Could you check a few things on this model? Use its own coordinates, in mm. Face numbers are marked on the shaded views. A direction names the side the tool comes from. Round coordinates to 2 decimals unless told otherwise and drop trailing zeros. Loops run counter-clockwise (first coordinate to the right, second up) from the corner with the lowest first, then second, coordinate; pieces in that order, holes last. Notation, with made-up numbers: M 27,11.25 L 78,11.25 A25 cw 78,23.25 Z; hole C 56.25,-19 d3. An arc over 180 degrees is marked long. Answer in a Markdown table with one row per item.
```python
from build123d import *

# Parameters (mm, degrees)
F1_DEPTH = 96
F2_R     = 7.5
F3_DEPTH = 30
F4_R     = 6
F5_DEPTH = 3
F6_R     = 6
F7_DEPTH = 3


with BuildPart() as f1:
    # F0 (on Top) → F1 (new body)
    with BuildSketch(Plane.XY):
        with BuildLine():
            ThreePointArc((0, -10), (-2.928932, -2.928932), (-10, 0))
            Line((-10, 0), (-97, 0))
            ThreePointArc((-97, 0), (-104.071068, -2.928932), (-107, -10))
            Line((-107, -10), (-107, -97))
            ThreePointArc((-107, -97), (-104.071068, -104.071068), (-97, -107))
            Line((-97, -107), (-10, -107))
            ThreePointArc((-10, -107), (-2.928932, -104.071068), (0, -97))
            Line((0, -97), (0, -10))
        make_face()
    extrude(amount=F1_DEPTH)

    # F2 (on face) → F3 (join)
    with BuildSketch(Plane(origin=(0, 0, 0), x_dir=(1, 0, 0), z_dir=(0, 0, -1))):
        with Locations((-53.5, 53.5)):
            Circle(F2_R)
    extrude(amount=F3_DEPTH)

    # F4 (on face) → F5 (cut)
    with BuildSketch(Plane.XY.offset(96)):
        with Locations((-94.5, -94.5)):
            Circle(F4_R)
        with Locations((-94.5, -12.5)):
            Circle(F4_R)
        with Locations((-12.5, -94.5)):
            Circle(F4_R)
        with Locations((-12.5, -12.5)):
            Circle(F4_R)
    extrude(amount=-F5_DEPTH, mode=Mode.SUBTRACT)

    # F6 (on face) → F7 (cut)
    with BuildSketch(Plane(origin=(0, 0, 0), x_dir=(1, 0, 0), z_dir=(0, 0, -1))):
        with Locations((-10, 97)):
            Circle(F6_R)
        with Locations((-10, 10)):
            Circle(F6_R)
        with Locations((-97, 97)):
            Circle(F6_R)
        with Locations((-97, 10)):
            Circle(F6_R)
    extrude(amount=-F7_DEPTH, mode=Mode.SUBTRACT)


solid = f1.part
```
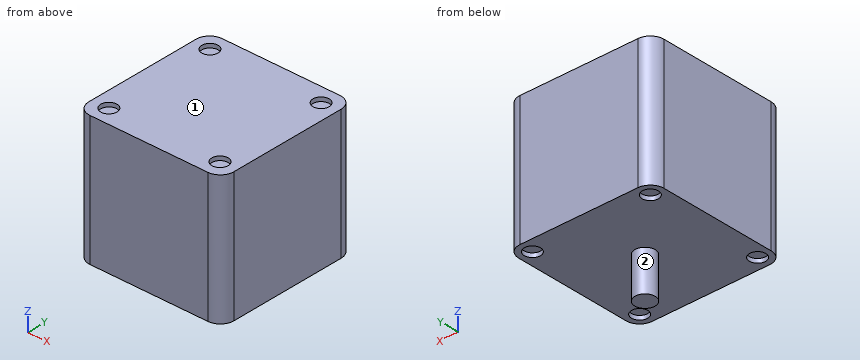
1) I want a section at B-B, the plane x = -53.5. Please give me the cut outline in (y, z).
Computed:
| item | result |
|---|---|
| outline | M -107,0 L -61,0 L -61,-30 L -46,-30 L -46,0 L 0,0 L 0,96 L -107,96 Z |
2) I want a section at A-A, the plane y = -58. Please give me the cut outline in (x, z), plus the area to 3 significant figures.
Computed:
| item | result |
|---|---|
| outline | M -107,0 L -59.5,0 L -59.5,-30 L -47.5,-30 L -47.5,0 L 0,0 L 0,96 L -107,96 Z |
| area | 10,600 mm² |
3) I want a section at C-C, the plane y = -84. Please give me the cut outline in (x, z).
Computed:
| item | result |
|---|---|
| outline | M -107,0 L 0,0 L 0,96 L -107,96 Z |
4) I need wall thicknesses on line 1 (Y direction, x = -94, z = 94); line 2 (Y direction, x = -97, z = 1). Which ranges of each line are inside material? Lowest first, please.
Computed:
| item | result |
|---|---|
| line 1 | y = -107 to -100.48, -88.52 to -18.48, -6.52 to 0 |
| line 2 | y = -107 to -103, -91 to -16, -4 to 0 |
5) Which directions (+Z, -Z, +X, -X, +Y, -Y) give clear straight access to the entire face, cutting with the end or side of a thin tool? Please do the marked faces 1 and 2.
Computed:
| item | result |
|---|---|
| face 1 | +Z, +X, -X, +Y, -Y |
| face 2 | -Z |
6) Will these pins go through, and if not, where does the flat tip stop? P1, Ø14, axis at x = -97, y = -97, coming from the -Z side; P2, Ø3.5, axis at x = -93, y = -92.5, coming from the +Z side; P3, Ø11, axis at x = -97, y = -10, coming from the -Z side.
Computed:
| item | result |
|---|---|
| P1 | stops at z = 0 |
| P2 | stops at z = 93 |
| P3 | stops at z = 3 |
